CAD build for the part. Positions are in the model's coordinates, mm. A direction names the side the tool comes from. Give positions to 0.01 mm unless a question says otherwise; leave off trailing zeros. Write each loop counter-clockwise with the first axis right and the second up, starting at its lowest first coordinate (ties: lowest second). Pieces come first, ordered by that corner, then holes. Notation, with made-up numbers: M 70.25,79 L 127.25,79 A21 ccw 127.25,112 Z; hole C 22.25,67.25 d3. An arc over 180 degrees is marked long. One line per question, with ' | ' between items. Start each with the question number.
1. Cut at C-C, the plane x = -4.75. Write the cut outline in (y, z), then the cut area to 3 significant figures.
2. Pull direction Y, two halves, no side cores. Call faces 1 (the face through (0, 0, 0)), 2 (the face through (0, 2.9, 2)), 3 (the face through (-6.35, 0, 2)): released by +Y, released by -Y, zero draft, split by the parting line, or undercut.
3. Which spindle directions (+Z, -Z, +X, -X, +Y, -Y) get a long thin tool onto all of the face, cutting with end or side? Do faces 4 (the face through (0, 0, 3.8)), 5 (the face through (0, -2.2, -1.6)). Say none if no direction does.
4. Flat gauge pin, fed straight in: pin 1 (0.6 mm diameter, centred on y = -2.5, z = -0.5, fed in from +X). Where does the tip first touch, or does it go through?
5. Wall check: L1, parallel to Y at x = 0.75, z = -1.5; L2, parallel to Z at x = -0.5, y = 2.4; L3, parallel to Z at x = 2.5, y = 1.3. Give the ranges that are in metal, low to high.
6. Cut at A-A, the plane z = -0.6. Write the cut outline in (x, y), then the cut area to 3 significant figures.
7. Cut at D-D, the plane y = -1. Write the cut outline in (x, z), then the cut area to 3 significant figures.
8. Cut at B-B, the plane y = -2.4. Write the cut outline in (x, z).
```python
from build123d import *

# Parameters (mm, degrees)
CROQUIS1_W              = 12.7
CROQUIS1_H              = 5.8
SALIENTE_EXTRUIR1_DEPTH = 3.8
CROQUIS2_W              = 3.7
CROQUIS2_H              = 0.7
SALIENTE_EXTRUIR2_DEPTH = 1.9
CROQUIS3_W              = 2
CROQUIS3_H              = 1.4
CORTAR_EXTRUIR1_DEPTH   = 2.95


with BuildPart() as part:
    # Croquis1 → Saliente-Extruir1 (new body)
    with BuildSketch(Plane.XY):
        Rectangle(CROQUIS1_W, CROQUIS1_H)
    extrude(amount=SALIENTE_EXTRUIR1_DEPTH)

    # Croquis2 → Saliente-Extruir2 (add)
    with BuildSketch(Plane.XY):
        with Locations((0, 2.55)):
            Rectangle(CROQUIS2_W, CROQUIS2_H)
        with Locations((0, -2.55)):
            Rectangle(CROQUIS2_W, CROQUIS2_H)
    extrude(amount=-SALIENTE_EXTRUIR2_DEPTH)

    # Croquis3 → Cortar-Extruir1 (cut, symmetric)
    with BuildSketch(Plane(origin=(0, 0, 0), x_dir=(1, 0, 0), z_dir=(0, 1, 0))):
        with Locations((0, 0.7)):
            Rectangle(CROQUIS3_W, CROQUIS3_H)
    extrude(amount=CORTAR_EXTRUIR1_DEPTH, both=True, mode=Mode.SUBTRACT)


solid = part.part
```
Here are the results:
1) outline: M -2.9,0 L 2.9,0 L 2.9,3.8 L -2.9,3.8 Z | area: 22.0 mm^2
2) face 1: undercut | face 2: released by +Y | face 3: zero draft
3) face 4: +Z, +X, -X, +Y, -Y | face 5: -Z, +X, -X
4) pin 1: x = 1.85
5) L1: -2.9 to -2.2, 2.2 to 2.9 | L2: -1.9 to -1.4, 0 to 3.8 | L3: 0 to 3.8
6) outline: M -1.85,-2.9 L -1,-2.9 L -1,-2.2 L -1.85,-2.2 Z; M -1.85,2.2 L -1,2.2 L -1,2.9 L -1.85,2.9 Z; M 1,-2.9 L 1.85,-2.9 L 1.85,-2.2 L 1,-2.2 Z; M 1,2.2 L 1.85,2.2 L 1.85,2.9 L 1,2.9 Z | area: 2.38 mm^2
7) outline: M -6.35,0 L 6.35,0 L 6.35,3.8 L -6.35,3.8 Z | area: 48.3 mm^2
8) outline: M -6.35,0 L -1.85,0 L -1.85,-1.9 L 1.85,-1.9 L 1.85,0 L 6.35,0 L 6.35,3.8 L -6.35,3.8 Z; hole M -1,-1.4 L 1,-1.4 L 1,0 L -1,0 Z
